Can you work these out from the drawing? Everything is in mm from the part's minimum corner. Round coordinates to 2 decimals unless told otherwise and drop trailing zeros. Use a Markdown table: item, result. Add a question column.
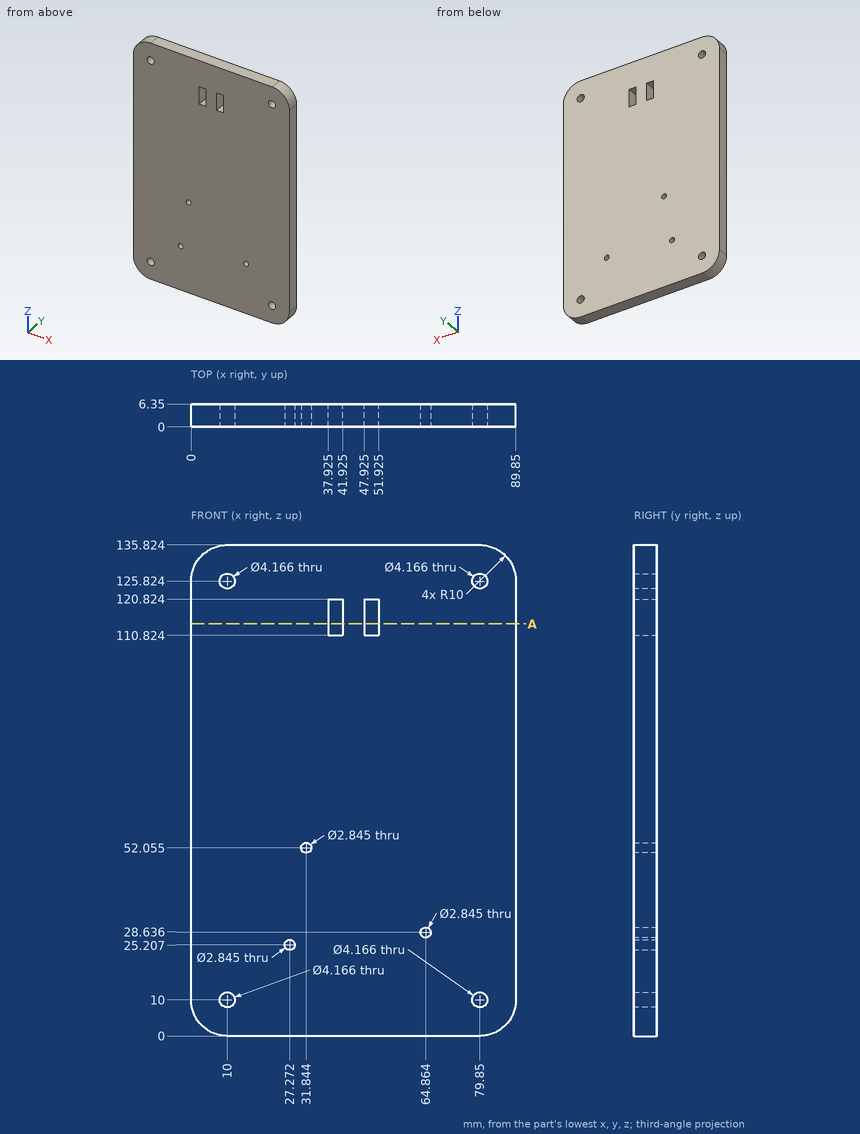
Item 1: Imagine slicing it at A-A on z = 114. Count the separate pieces of the cut face and the enclosed holes in it, plus the area to 3 significant figures.
Item 2: For pin 1 Ø3.5 at (x, z) = (64.864, 28.636) entering from +Y, with a flat end and sliding along its axis, tell me the tip position at first contact or that it passes through.
Item 3: I need wall thicknesses on probe 1 along Z at (x, y) = (79.85, 5.25); probe 2 along Z at (x, y) = (65, 5); probe 3 along Z at (x, y) = (5, 4.25) (1 decimal). Which ranges of each line are inside material? Lowest first, please. Write a range as from..to.
The answers:
| question | item | result |
|---|---|---|
| 1 | separate pieces | 3 |
| 1 | enclosed holes | 0 |
| 1 | area | 520 mm² |
| 2 | pin 1 | y = 6.35 |
| 3 | probe 1 | 0..7.92, 12.08..123.74, 127.91..135.82 |
| 3 | probe 2 | 0..27.22, 30.05..135.82 |
| 3 | probe 3 | 1.3..134.5 |
